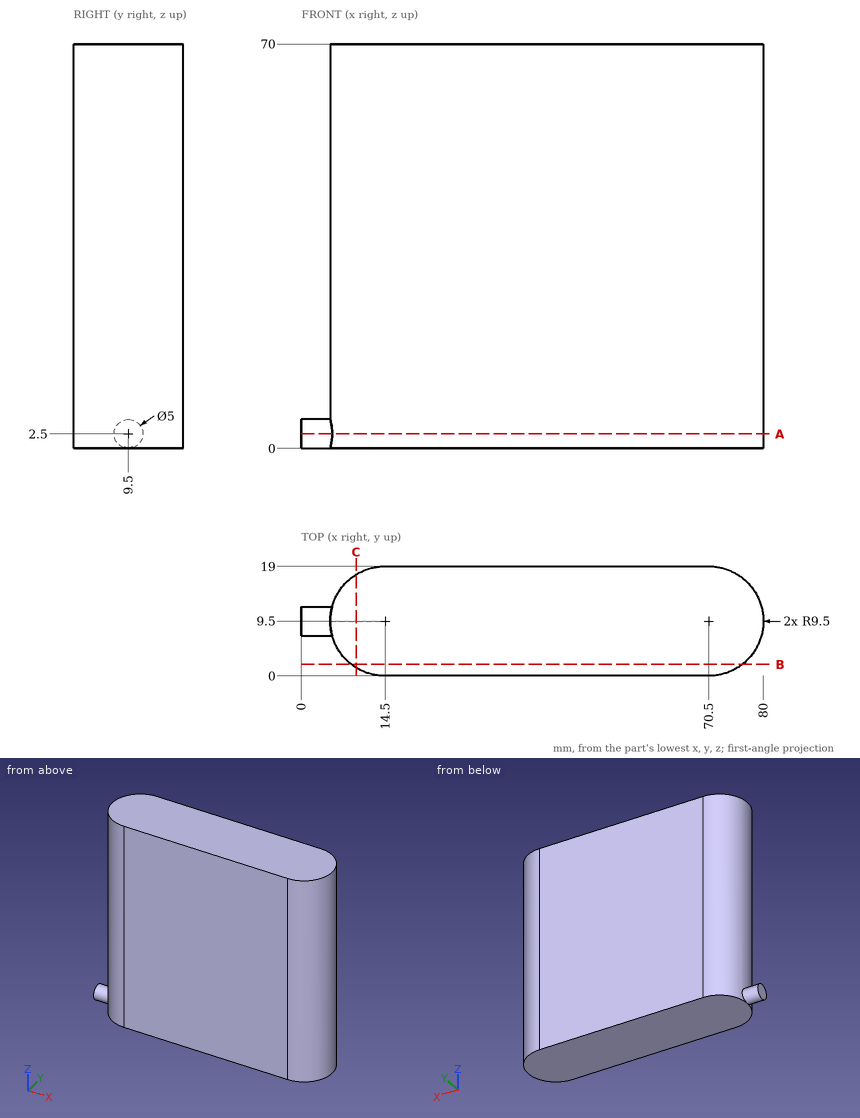
Part print with two shaded views. Sizes in mm from the minimum x, y, z corner. Round coordinates to 2 decimals unless told otherwise and drop trailing zeros. Loops run counter-clockwise (first coordinate to the right, second up) from the corner with the lowest first, then second, coordinate; pieces in that order, holes last. Notation, with made-up numbers: (-12.5, 73) - (9.5, 73) arc R11 ccw to (9.5, 93) - close; hole circle Ø5 at (-16.5, 44.5). An arc over 180 degrees is marked (long way). Answer as a JSON object with one key per item and string values.
Item 1: Band-saw the part on C-C on x = 9.5. List the corners of the cut face in (y, z), plus the area to 3 significant figures.
Output:
{"outline": "(1.42, 0) - (17.58, 0) - (17.58, 70) - (1.42, 70) - close", "area": "1,130 mm2"}
Item 2: Band-saw the part on B-B on y = 2. List the corners of the cut face in (x, z).
Output:
{"outline": "(8.67, 0) - (76.33, 0) - (76.33, 70) - (8.67, 70) - close"}
Item 3: Wall check: L1, parallel to Z at x = 3, y = 9.75; L2, parallel to Y at x = 8, z = 23.5; L3, parallel to X at y = 1.75, z = 49.5. Give the ranges that are in metal, low to high.
Output:
{"L1": "0.01 to 4.99", "L2": "2.57 to 16.43", "L3": "9.01 to 75.99"}
Item 4: Band-saw the part on A-A on z = 2.5. List the corners of the cut face in (x, y).
Output:
{"outline": "(0, 7) - (5.33, 7) arc R9.5 ccw to (14.5, 0) - (70.5, 0) arc R9.5 ccw to (70.5, 19) - (14.5, 19) arc R9.5 ccw to (5.33, 12) - (0, 12) - close"}
Item 5: Pin check, flat tips, straight feed: pin 1 (5 mm diameter, centred on y = 14, z = 8.5, fed in from +X); pin 2 (1.5 mm diameter, centred on y = 17, z = 34.5, fed in from +X); pin 3 (5 mm diameter, centred on y = 15, z = 19, fed in from -X). Stop position of each tip, or through.
Output:
{"pin 1": "x = 79.79", "pin 2": "x = 77.18", "pin 3": "x = 5.49"}
